from build123d import *

# Parameters (mm, degrees)
EXTRUDE_1_DEPTH     = 2
SKETCH_2_R          = 0.75
CUT_EXTRUDE_1_DEPTH = 36.34566511
FILLET_1_R          = 1


with BuildPart() as part:
    # 草图1 → 凸台-拉伸1 (new body)
    with BuildSketch(Plane.XY):
        with BuildLine():
            Line((4.139173101, 1.990268069), (-34.5, 7.420649709))
            Line((-34.5, 7.420649709), (-34.5, 0))
            Line((-34.5, 0), (-32, 0))
            Line((-32, 0), (-32, -3))
            Line((-32, -3), (-22, -3))
            Line((-22, -3), (-22, 0))
            Line((-22, 0), (-10, 0))
            Line((-10, 0), (-10, -3))
            Line((-10, -3), (0, -3))
            Line((0, -3), (0, 0))
            Line((0, 0), (4, 0))
            ThreePointArc((4, 0), (4.99756405, 0.930243526), (4.139173101, 1.990268069))
        make_face()
    extrude(amount=EXTRUDE_1_DEPTH)

    # 草图2 → 切除-拉伸1 (cut, through all)
    with BuildSketch(Plane.XY.offset(2)):
        with Locations((-32.75, 0)):
            Circle(SKETCH_2_R)
        with Locations((-21.25, 0)):
            Circle(SKETCH_2_R)
        with Locations((-10.75, 0)):
            Circle(SKETCH_2_R)
        with Locations((0.75, 0)):
            Circle(SKETCH_2_R)
    extrude(amount=-CUT_EXTRUDE_1_DEPTH, mode=Mode.SUBTRACT)

    # 圆角1
    fillet_1_edges = [part.edges().sort_by_distance(p)[0] for p in [
        (0, -3, 1),
        (-10, -3, 1),
        (-22, -3, 1),
        (-32, -3, 1),
    ]]
    fillet(fillet_1_edges, radius=FILLET_1_R)


solid = part.part
Could you check a few things on this model? Use its own coordinates, in mm. A direction names the side the tool comes from. Round coordinates to 2 decimals unless told otherwise and drop trailing zeros. Order: outer loops, then holes, each group sorted by start corner. A loop starts at its lowest first (then second) coordinate and runs counter-clockwise, first axis right, second up.
(1) Imagine slicing it at B-B (x = -10.75). Write out the boundary of the cut face in (y, z).
Response values:
outline: (0.75, 0) - (4.08, 0) - (4.08, 2) - (0.75, 2) - close
(2) Imagine slicing it at C-C (y = 5.25). Write out the boundary of the cut face in (x, z).
Response values:
outline: (-34.5, 0) - (-19.06, 0) - (-19.06, 2) - (-34.5, 2) - close
(3) If we mould it in two halves opening along X, with no side actions, what happens to faces 1 (the flat face through (-34.5, 4, 1)), 2 (the cylindrical face through (-10.73, 0.75, 1.01)), 3 (the flat face through (-14.91, 4.667, 0.986)), 4 (the flat face through (-34, 0, 1))? For each: released by +X, released by -X, zero draft, split by the parting line, or undercut.
Response values:
face 1: released by -X
face 2: undercut
face 3: released by +X
face 4: zero draft
(4) Please list where these lines run through material, in increasing order: line 1 along X through (y, z) = (-0.5, 1.75); line 2 along X through (y, z) = (0.25, 1.8); line 3 along Y through (x, z) = (-24, 0.35).
Response values:
line 1: x = -32 to -22, -10 to 0
line 2: x = -34.5 to -33.46, -32.04 to -21.96, -20.54 to -11.46, -10.04 to 0.04, 1.46 to 4.66
line 3: y = -3 to 5.94
(5) I'm going to push flat-ended pins straight in: pin 1 (0.6 mm diameter, centred on y = -0.5, z = 1, fed in from -X); pin 2 (0.5 mm diameter, centred on x = -34, z = 1, fed in from -Y); pin 3 (0.6 mm diameter, centred on y = -0.5, z = 1, fed in from +X). Where does each tip first touch, or does it pass through?
Response values:
pin 1: stops at x = -32
pin 2: stops at y = 0
pin 3: stops at x = 0
(6) Which directions (+Z, -Z, +X, -X, +Y, -Y) give clear straight access to the entire face, cutting with the end or side of a thin tool? Please do faces 5 (the cylindrical face through (-22.285, -2.699, 1.014)), 6 (the flat face through (3, 0, 1)), 7 (the flat face through (-32, -1, 1)).
Response values:
face 5: +Z, -Z, -Y
face 6: +Z, -Z, +X, -Y
face 7: +Z, -Z, -X, -Y
(7) Imagine slicing it at A-A (z = 1). Write out the boundary of the cut face in (x, y), plus the area to 3 significant figures.
Response values:
outline: (-34.5, 0) - (-33.5, 0) arc R0.75 cw to (-32, 0) - (-32, -2) arc R1 ccw to (-31, -3) - (-23, -3) arc R1 ccw to (-22, -2) - (-22, 0) arc R0.75 cw to (-20.5, 0) - (-11.5, 0) arc R0.75 cw to (-10, 0) - (-10, -2) arc R1 ccw to (-9, -3) - (-1, -3) arc R1 ccw to (0, -2) - (0, 0) arc R0.75 cw to (1.5, 0) - (4, 0) arc R1 ccw to (4.14, 1.99) - (-34.5, 7.42) - close
area: 239 mm2
